```python
from build123d import *

# Parameters (mm, degrees)
ESQUISSE3_W                       = 60.424633044
ESQUISSE3_H                       = 3.5
ENL_V_MAT_EXTRU_3_DEPTH           = 15
ENL_V_MAT_EXTRU_3_DRAFT           = 1
ENL_V_MAT_EXTRU_3_PROFILE_2_DEPTH = 15
ENL_V_MAT_EXTRU_3_PROFILE_2_DRAFT = 1
ESQUISSE3_W_2                     = 42
ESQUISSE3_H_2                     = 3.2
ENL_V_MAT_EXTRU_3_PROFILE_3_DEPTH = 15
ENL_V_MAT_EXTRU_3_PROFILE_3_DRAFT = 1
CONG_1_R                          = 3


with BuildPart() as part:
    # Esquisse1 → Lissage1 section 0
    with BuildSketch(Plane.XY):
        with BuildLine():
            Line((-23, 27.75), (23, 27.75))
            Line((23, 27.75), (23, -27.75))
            Line((23, -27.75), (-23, -27.75))
            Line((-23, -27.75), (-23, 27.75))
        make_face()
    # Esquisse2 → Lissage1 section 1
    with BuildSketch(Plane.XY.offset(-20)):
        with BuildLine():
            Line((-26, 30.25), (23, 30.25))
            Line((23, 30.25), (23, -30.25))
            Line((23, -30.25), (-26, -30.25))
            Line((-26, -30.25), (-26, 30.25))
        make_face()
    loft()


with BuildPart() as enl_v_mat_extru_3_tool:
    # Esquisse3 → Enlèv. mat.-Extru.3 (with draft: the straight prism first)
    with BuildSketch(Plane.XY.offset(-20)):
        with Locations((-0.930868515, 2.5)):
            Rectangle(ESQUISSE3_W, ESQUISSE3_H)
    extrude(amount=ENL_V_MAT_EXTRU_3_DEPTH)
    # Enlèv. mat.-Extru.3: the draft: its side faces are tilted about the plane it starts from
    enl_v_mat_extru_3_sides = [enl_v_mat_extru_3_tool.faces().sort_by_distance(p)[0] for p in [
        (-0.930868515, 0.75, -12.5),
        (29.281448007, 2.5, -12.5),
        (-0.930868515, 4.25, -12.5),
        (-31.143185037, 2.5, -12.5),
    ]]
    draft(enl_v_mat_extru_3_sides, Plane.XY.offset(-20), ENL_V_MAT_EXTRU_3_DRAFT)


with BuildPart() as part_1:
    add(part.part)

    # Enlèv. mat.-Extru.3: cut by enl_v_mat_extru_3_tool
    add(enl_v_mat_extru_3_tool.part, mode=Mode.SUBTRACT)


with BuildPart() as enl_v_mat_extru_3_profile_2_tool:
    # Esquisse3 → Enlèv. mat.-Extru.3 profile 2 (with draft: the straight prism first)
    with BuildSketch(Plane.XY.offset(-20)):
        with Locations((-2.538455813, 18)):
            Rectangle(ESQUISSE3_W, ESQUISSE3_H)
    extrude(amount=ENL_V_MAT_EXTRU_3_PROFILE_2_DEPTH)
    # Enlèv. mat.-Extru.3 profile 2: the draft: its side faces are tilted about the plane it starts from
    enl_v_mat_extru_3_profile_2_sides = [enl_v_mat_extru_3_profile_2_tool.faces().sort_by_distance(p)[0] for p in [
        (-2.538455813, 16.25, -12.5),
        (27.673860709, 18, -12.5),
        (-2.538455813, 19.75, -12.5),
        (-32.750772335, 18, -12.5),
    ]]
    draft(enl_v_mat_extru_3_profile_2_sides, Plane.XY.offset(-20), ENL_V_MAT_EXTRU_3_PROFILE_2_DRAFT)


with BuildPart() as part_2:
    add(part_1.part)

    # Enlèv. mat.-Extru.3 profile 2: cut by enl_v_mat_extru_3_profile_2_tool
    add(enl_v_mat_extru_3_profile_2_tool.part, mode=Mode.SUBTRACT)


with BuildPart() as enl_v_mat_extru_3_profile_3_tool:
    # Esquisse3 → Enlèv. mat.-Extru.3 profile 3 (with draft: the straight prism first)
    with BuildSketch(Plane.XY.offset(-20)):
        with Locations((0, -15.85)):
            Rectangle(ESQUISSE3_W_2, ESQUISSE3_H_2)
    extrude(amount=ENL_V_MAT_EXTRU_3_PROFILE_3_DEPTH)
    # Enlèv. mat.-Extru.3 profile 3: the draft: its side faces are tilted about the plane it starts from
    enl_v_mat_extru_3_profile_3_sides = [enl_v_mat_extru_3_profile_3_tool.faces().sort_by_distance(p)[0] for p in [
        (0, -17.45, -12.5),
        (21, -15.85, -12.5),
        (0, -14.25, -12.5),
        (-21, -15.85, -12.5),
    ]]
    draft(enl_v_mat_extru_3_profile_3_sides, Plane.XY.offset(-20), ENL_V_MAT_EXTRU_3_PROFILE_3_DRAFT)


with BuildPart() as part_3:
    add(part_2.part)

    # Enlèv. mat.-Extru.3 profile 3: cut by enl_v_mat_extru_3_profile_3_tool
    add(enl_v_mat_extru_3_profile_3_tool.part, mode=Mode.SUBTRACT)

    # Congé1
    cong_1_edges = [part_3.edges().sort_by_distance(p)[0] for p in [
        (-24.5, 29, -10),
        (-24.5, -29, -10),
    ]]
    fillet(cong_1_edges, radius=CONG_1_R)


solid = part_3.part
```
Design review of the part built by this model. Coordinates are the model's own, in mm. A direction names the side the tool comes from. Give positions to 0.01 mm unless a question says otherwise; leave off trailing zeros. Answer in a Markdown table with one row per item.
(1) Mouldability with a two-part tool opening along Y and no side actions: class faces 3 (the flat face through (0, -16, -5)), 4 (the flat face through (-2, 26, -20)) as +Y half, -Y half, draft (parallel to the pull), parting line (faces both ways), or undercut.
Results:
| item | result |
|---|---|
| face 3 | undercut |
| face 4 | draft |
(2) Clearance check with flat-ended pins moving along their axes: pin 1 (1.5 mm diameter, centred on x = -8.5, y = 2.5, fed in from -Z); pin 2 (1 mm diameter, centred on y = -9.5, z = -11.5, fed in from -X); pin 3 (5 mm diameter, centred on y = -3.5, z = -11.5, fed in from -X). State where each tip first meets the part, or that it passes through.
Results:
| item | result |
|---|---|
| pin 1 | z = -5 |
| pin 2 | x = -24.8 |
| pin 3 | x = -25.1 |
(3) For faces 1 (the flat face through (-1, -14, -20)), 2 (the flat face through (-1, 3, -5)), list the 3-axis set-ups (+Z, -Z, +X, -X, +Y, -Y) from which the entire face can be reached by the end or side of a thin tool; tool diameter is ignored.
Results:
| item | result |
|---|---|
| face 1 | -Z, +X, -X, +Y, -Y |
| face 2 | -Z, +X, -X |
(4) Consider section A-A (z = -6). Count the separate pieces of the cut face and the enclosed holes in it, then the cut area to 3 significant figures.
Results:
| item | result |
|---|---|
| separate pieces | 3 |
| enclosed holes | 1 |
| area | 2,270 mm2 |
(5) To check wall thickness, follow probe 1 along Y at (x, z) = (-1, -16.75); probe 2 along Y at (x, z) = (4, -10.5); probe 3 along X at (y, z) = (-17, -5.25). State the ranges of each line that lie inside material, in increasing order.
Results:
| item | result |
|---|---|
| probe 1 | -29.84 to -17.39, -14.31 to 0.81, 4.19 to 16.31, 19.69 to 29.84 |
| probe 2 | -29.06 to -17.28, -14.42 to 0.92, 4.08 to 16.42, 19.58 to 29.06 |
| probe 3 | -23.79 to -20.74, 20.74 to 23 |
